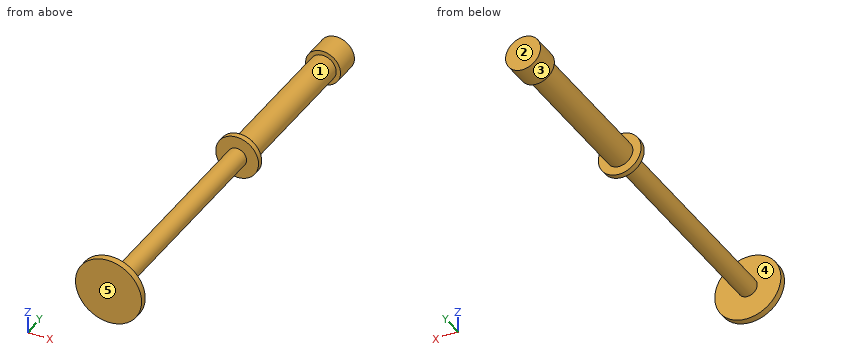
```python
from build123d import *

# Parameters (mm, degrees)
F0_R     = 5.55
F1_DEPTH = 8
F2_R     = 4.175
F3_DEPTH = 55.7
F4_R     = 6.8
F5_DEPTH = 1.8
F6_R     = 3
F7_DEPTH = 72
F8_R     = 10.5
F9_DEPTH = 2.1


with BuildPart() as f1:
    # F0 (on Front) → F1 (new body)
    with BuildSketch(Plane.XZ):
        Circle(F0_R)
    extrude(amount=F1_DEPTH)

    # F2 (on Front) → F3 (join)
    with BuildSketch(Plane.XZ):
        Circle(F2_R)
    extrude(amount=F3_DEPTH)

    # F4 (on face) → F5 (join)
    with BuildSketch(Plane.XZ.offset(55.7)):
        Circle(F4_R)
    extrude(amount=F5_DEPTH)

    # F6 (on face) → F7 (join)
    with BuildSketch(Plane.XZ.offset(57.5)):
        Circle(F6_R)
    extrude(amount=F7_DEPTH)

    # F8 (on face) → F9 (join)
    with BuildSketch(Plane.XZ.offset(129.5)):
        Circle(F8_R)
    extrude(amount=F9_DEPTH)


solid = f1.part
```
CAD build for the part. Positions are in the model's coordinates, mm. Face numbers are marked on the shaded views. A direction names the side the tool comes from. Coordinates: 2 decimals unless noted, no trailing zeros. Order: outer loops, then holes, each group sorted by start corner. A loop starts at its lowest first (then second) coordinate and runs counter-clockwise, first axis right, second up. Notation, with made-up numbers: (6.25, 81.25) - (38.25, 81.25) arc R14 cw to (38.25, 100.25) - close; hole circle Ø9 at (-29, -3). An arc over 180 degrees is marked (long way). Use a Markdown table: item, result. Add a question column.
(1) Pull direction Y, two halves, no side cores. Call the marked faces 1, 2 and 3: +Y half, -Y half, draft (parallel to the pull), parting line (faces both ways), or undercut.
(2) Drill centre lines: line 1 along Y through (x, z) = (0.5, -6); line 2 along Y through (x, z) = (0.75, -7.5); line 3 along Z through (x, y) = (-2.5, -13). Where is each one in solid material? Low to high. Write a range as [from, to].
(3) Saw through at A-A (z = 0). Give the cut face in (x, y) (3 decimals), then the cut area to 3 significant figures.
(4) Saw through at C-C (y = -79). Give the cut face in (x, z).
(5) Which spindle directions (+Z, -Z, +X, -X, +Y, -Y) get a long thin tool onto all of the face, cutting with end or side? Do the marked faces 4 and 5. Say none if no direction does.
(6) Flat gauge pins, fed straight in: pin 1 (3 mm diameter, centred on x = -1, y = -14.5, fed in from -Z) (3 decimals); pin 2 (6 mm diameter, centred on x = 5, y = -18, fed in from +Z); pin 3 (10 mm diameter, centred on y = -75, z = 2.5, fed in from +X). Where does each tip first touch, or does it go through?
(7) Saw through at B-B (x = 0). Give the cut face in (y, z) (3 decimals).
(8) Saw through at D-D (y = -12.5). Give the cut face in (x, z) (3 decimals), then the cut area to 3 significant figures.
Solved:
| question | item | result |
|---|---|---|
| 1 | face 1 | undercut |
| 1 | face 2 | +Y half |
| 1 | face 3 | draft |
| 2 | line 1 | y = [-131.6, -129.5], [-57.5, -55.7] |
| 2 | line 2 | y = [-131.6, -129.5] |
| 2 | line 3 | z = [-3.34, 3.34] |
| 3 | outline | (-10.5, -131.6) - (10.5, -131.6) - (10.5, -129.5) - (3, -129.5) - (3, -57.5) - (6.8, -57.5) - (6.8, -55.7) - (4.175, -55.7) - (4.175, -8) - (5.55, -8) - (5.55, 0) - (-5.55, 0) - (-5.55, -8) - (-4.175, -8) - (-4.175, -55.7) - (-6.8, -55.7) - (-6.8, -57.5) - (-3, -57.5) - (-3, -129.5) - (-10.5, -129.5) - close |
| 3 | area | 988 mm² |
| 4 | outline | circle Ø6 at (0, 0) |
| 5 | face 4 | none |
| 5 | face 5 | +Z, -Z, +X, -X, -Y |
| 6 | pin 1 | stops at z = -4.175 |
| 6 | pin 2 | stops at z = 3.66 |
| 6 | pin 3 | stops at x = 3 |
| 7 | outline | (-131.6, -10.5) - (-129.5, -10.5) - (-129.5, -3) - (-57.5, -3) - (-57.5, -6.8) - (-55.7, -6.8) - (-55.7, -4.175) - (-8, -4.175) - (-8, -5.55) - (0, -5.55) - (0, 5.55) - (-8, 5.55) - (-8, 4.175) - (-55.7, 4.175) - (-55.7, 6.8) - (-57.5, 6.8) - (-57.5, 3) - (-129.5, 3) - (-129.5, 10.5) - (-131.6, 10.5) - close |
| 8 | outline | circle Ø8.35 at (0, 0) |
| 8 | area | 54.8 mm² |
